Source: CAD feature listing. Evaluate the final solid. Frame: model axes, mm. A direction names the side the tool comes from. Round coordinates to 2 decimals unless told otherwise and drop trailing zeros. Write each loop counter-clockwise with the first axis right and the second up, starting at its lowest first coordinate (ties: lowest second). Pieces come first, ordered by that corner, then holes. Notation, with made-up numbers: M -23,18 L -17,18 A19 cw -17,32 Z; hole C 54,69 d2. An arc over 180 degrees is marked long. Use a Markdown table: item, result.
```python
from build123d import *

# Parameters (mm, degrees)
F0_R     = 5
F1_DEPTH = 7.5
F2_R     = 10
F3_DEPTH = 200


with BuildPart() as f1:
    # F0 (on Top) → F1 (new body, symmetric)
    with BuildSketch(Plane.XY):
        with BuildLine():
            Line((-10, -25), (10, -25))
            Line((10, -25), (10, 25))
            ThreePointArc((10, 25), (0, 35), (-10, 25))
            Line((-10, 25), (-10, -25))
        make_face()
        with Locations((0, 25)):
            Circle(F0_R, mode=Mode.SUBTRACT)
    extrude(amount=F1_DEPTH, both=True)

    # F2 (on face) → F3 (join)
    with BuildSketch(Plane.XZ.offset(25)):
        Circle(F2_R)
    extrude(amount=F3_DEPTH)


solid = f1.part
```
Q1. Line query: L1, parallel to Y at x = 0, z = -3.25; L2, parallel to Z at x = -6.75, y = 17; L3, parallel to Y at x = 2.75, z = 6.25. Output: solid intervals per line, ascending.
Results are:
| item | result |
|---|---|
| L1 | -225 to 20, 30 to 35 |
| L2 | -7.5 to 7.5 |
| L3 | -225 to 20.82, 29.18 to 34.61 |
Q2. First-contact query: pin 1 Ø10 at (x, z) = (-6.5, -7.5) entering from +Y; pin 2 Ø6 at (x, y) = (-4.5, -108.5) entering from -Z; pin 3 Ø2 at (y, z) = (-59, 7.5) entering from -X; pin 4 Ø6 at (x, y) = (0, 25) entering from -Z. Flat tips, straight axial feed; report the tip coordinate or a pass-through.
Results are:
| item | result |
|---|---|
| pin 1 | y = 34.89 |
| pin 2 | z = -9.89 |
| pin 3 | x = -7.6 |
| pin 4 | through |
Q3. Section C-C on y = -188.5. Return loops of the section in (x, z), plus the area to 3 significant figures.
Results are:
| item | result |
|---|---|
| outline | C 0,0 d20 |
| area | 314 mm^2 |
Q4. Section A-A on x = 0. Return loops of the section in (y, z), plus the area to 3 significant figures.
Results are:
| item | result |
|---|---|
| outline | M -225,-10 L -25,-10 L -25,-7.5 L 20,-7.5 L 20,7.5 L -25,7.5 L -25,10 L -225,10 Z; M 30,-7.5 L 35,-7.5 L 35,7.5 L 30,7.5 Z |
| area | 4,750 mm^2 |
Q5. Section B-B on z = -2.25. Return loops of the section in (x, y).
Results are:
| item | result |
|---|---|
| outline | M -10,-25 L -9.74,-25 L -9.74,-225 L 9.74,-225 L 9.74,-25 L 10,-25 L 10,25 A10 ccw -10,25 Z; hole C 0,25 d10 |
Q6. Mould query, pull axis Y, two halves, no side actions, for faces 1 (the cylindrical face through (0, 35, 0)), 2 (the cylindrical face through (-1.08, 20.12, -0.11)), 3 (the flat face through (10, 0, 0)). Classes: +Y half, -Y half, draft (parallel to the pull), parting line (faces both ways), or undercut.
Results are:
| item | result |
|---|---|
| face 1 | +Y half |
| face 2 | undercut |
| face 3 | draft |
Q7. Reachability of faces 4 (the flat face through (0, 5, -7.5)), 5 (the flat face through (0, 5, 7.5)), 6 (the cylindrical face through (-2.17, -123.6, -9.76)), 7 (the flat face through (-10, 0, 0)) from +Z, -Z, +X, -X, +Y, -Y: full face, straight path, thin tool, end or side. Return the list, or none.
Results are:
| item | result |
|---|---|
| face 4 | -Z, +X, -X, +Y |
| face 5 | +Z, +X, -X, +Y |
| face 6 | -Y |
| face 7 | +Z, -Z, -X, +Y, -Y |
Q8. Section D-D on y = -8. Return loops of the section in (x, z), plus the area to 3 significant figures.
Results are:
| item | result |
|---|---|
| outline | M -10,-7.5 L 10,-7.5 L 10,7.5 L -10,7.5 Z |
| area | 300 mm^2 |
